from build123d import *

# Parameters (mm, degrees)
F1_DEPTH = 9.9568
F2_R     = 3.175
F3_DEPTH = 2.921
F4_R     = 3.175
F5_DEPTH = 2.921
F6_R     = 3.175
F7_DEPTH = 12.7
F8_SIZE  = 0.254


with BuildPart() as f1:
    # F0 (on Top) → F1 (new body)
    with BuildSketch(Plane.XY):
        with BuildLine():
            Line((-6.223, 7.211095), (-6.223, -7.211095))
            ThreePointArc((-6.223, -7.211095), (9.525, 0), (-6.223, 7.211095))
        make_face()
    extrude(amount=F1_DEPTH)

    # F2 (on face) → F3 (join)
    with BuildSketch(Plane(origin=(0, 0, 0), x_dir=(1, 0, 0), z_dir=(0, 0, -1))):
        Circle(F2_R)
    extrude(amount=F3_DEPTH)

    # F4 (on face) → F5 (join)
    with BuildSketch(Plane.XY.offset(9.9568)):
        Circle(F4_R)
    extrude(amount=F5_DEPTH)

    # F6 (on face) → F7 (cut)
    with BuildSketch(Plane(origin=(-6.223, 0, 0), x_dir=(0, -1, 0), z_dir=(-1, 0, 0))):
        with Locations((0, 4.9784)):
            Circle(F6_R)
    extrude(amount=-F7_DEPTH, mode=Mode.SUBTRACT)

    # F8
    f8_edges = [f1.edges().sort_by_distance(p)[0] for p in [
        (-3.175, 0, -2.921),
        (9.525, 0, 9.9568),
        (9.525, 0, 0),
        (-3.175, 0, 12.8778),
    ]]
    chamfer(f8_edges, length=F8_SIZE)


solid = f1.part
Work out the finished part from the listing and answer in its coordinate system (mm). A direction names the side the tool comes from. Give positions to 0.01 mm unless a question says otherwise; leave off trailing zeros. Order: outer loops, then holes, each group sorted by start corner. A loop starts at its lowest first (then second) coordinate and runs counter-clockwise, first axis right, second up. Notation, with made-up numbers: (59.25, -16) -> (87.25, -16) arc R26 cw to (87.25, 22) -> close; hole circle Ø11 at (-7, 68.5). An arc over 180 degrees is marked (long way). One line per item, written item: value.
Item 1: Find section A-A, the plane x = 0. Give the vertices of the cut face in (y, z) (3 decimals), plus the area to 3 significant figures.
Answer sheet:
outline: (-9.525, 0.254) -> (-9.271, 0) -> (-3.175, 0) -> (-3.175, -2.667) -> (-2.921, -2.921) -> (2.921, -2.921) -> (3.175, -2.667) -> (3.175, 0) -> (9.271, 0) -> (9.525, 0.254) -> (9.525, 9.703) -> (9.271, 9.957) -> (3.175, 9.957) -> (3.175, 12.624) -> (2.921, 12.878) -> (-2.921, 12.878) -> (-3.175, 12.624) -> (-3.175, 9.957) -> (-9.271, 9.957) -> (-9.525, 9.703) -> close; hole circle Ø6.35 at (0, 4.978)
area: 195 mm²
Item 2: A tool of negligible diameter and unlimited length cuts with its end or side. For faces 4 (the cylindrical face through (-0.69, 3.1, -1.31)), 5 (the cylindrical face through (9.52, -0.3, 4.91)), 6 (the flat face through (6.477, 0, 5)), 7 (the cylindrical face through (-0.69, -3.1, 11.27)), from which of +Z, -Z, +X, -X, +Y, -Y can it reach the whole face along a straight path? Write none if from no direction.
Answer sheet:
face 4: -Z
face 5: +Z, -Z
face 6: -X
face 7: +Z
Item 3: Straight lines are drawn through the part: probe 1 along Z at (x, y) = (-1.25, 0); probe 2 along Y at (x, z) = (-0.75, 5.25); probe 3 along Z at (x, y) = (0.75, 0.5). For each, find the intervals that lie inside material, in ascending order.
Answer sheet:
probe 1: -2.92 to 1.8, 8.15 to 12.88
probe 2: -9.5 to -3.16, 3.16 to 9.5
probe 3: -2.92 to 1.84, 8.11 to 12.88
Item 4: Determine the mould class of faces 1 (the cylindrical face through (0.038, 0.413, 8.126)), 2 (the flat face through (0, 0, -2.921)), 3 (the conical face through (9.391, -0.303, 9.832)) for opening direction Y: released by +Y, released by -Y, zero draft, split by the parting line, or undercut.
Answer sheet:
face 1: undercut
face 2: zero draft
face 3: split by the parting line
Item 5: Find section B-B, the plane y = 0. Give the vertices of the cut face in (x, z) (3 decimals).
Answer sheet:
outline: (-6.223, 0) -> (-3.175, 0) -> (-3.175, -2.667) -> (-2.921, -2.921) -> (2.921, -2.921) -> (3.175, -2.667) -> (3.175, 0) -> (9.271, 0) -> (9.525, 0.254) -> (9.525, 9.703) -> (9.271, 9.957) -> (3.175, 9.957) -> (3.175, 12.624) -> (2.921, 12.878) -> (-2.921, 12.878) -> (-3.175, 12.624) -> (-3.175, 9.957) -> (-6.223, 9.957) -> (-6.223, 8.153) -> (6.477, 8.153) -> (6.477, 1.803) -> (-6.223, 1.803) -> close
Item 6: Find section C-C, the plane z = -0.75. Give the vertices of the cut face in (x, y) (3 decimals).
Answer sheet:
outline: circle Ø6.35 at (0, 0)
Item 7: Flat-ended cylindrical pins translate along their axes: P1, Ø1.5, axis at x = 7, y = 4.5, coming from the -Z side; P2, Ø1.5, axis at y = -2, z = 5.5, coming from the +X side; P3, Ø5.5, axis at y = 0, z = 4.98, coming from the -X side. Find the tip coordinate at first contact, or state that the pin passes through.
Answer sheet:
P1: z = 0
P2: x = 9.44
P3: x = 6.48
Item 8: Find section D-D, the plane z = 4. Give the vertices of the cut face in (x, y) (3 decimals).
Answer sheet:
outline: (-6.223, -7.211) arc R9.525 ccw (long way) to (-6.223, 7.211) -> (-6.223, 3.02) -> (6.477, 3.02) -> (6.477, -3.02) -> (-6.223, -3.02) -> close
